Could you check a few things on this model? Use its own coordinates, in mm. A direction names the side the tool comes from. Coordinates: 2 decimals unless noted, no trailing zeros. Loops run counter-clockwise (first coordinate to the right, second up) from the corner with the lowest first, then second, coordinate; pieces in that order, holes last. Notation, with made-up numbers: (51, 45) - (96, 45) arc R25 ccw to (96, 75) - close; hole circle Ø4 at (19, 74). An arc over 180 degrees is marked (long way). One line per question, with ' | ' between items. Start each with the question number.
1. I want a section at C-C, the plane z = 696.5. Write out the boundary of the cut face in (x, y).
2. I'm going to push flat-ended pins straight in: P1, Ø2, axis at x = 12.5, y = 1.5, coming from the +Z side; P2, Ø8, axis at x = -11.5, y = -1, coming from the +Z side. Where does each tip first touch, or does it pass through?
3. I want a section at A-A, the plane x = 4.5. Write out the boundary of the cut face in (y, z).
4. Please list where these lines run through material, in increasing order: L1, parallel to Y at x = -1, z = 61; L2, parallel to Y at x = -13, z = 205. Write a range as [from, to].
5. Which directions (+Z, -Z, +X, -X, +Y, -Y) give clear straight access to the entire face, cutting with the end or side of a thin tool? Please do faces 1 (the flat face through (-14.5, 0, 360)), 2 (the flat face through (17.5, 0, 360)).
6. I want a section at B-B, the plane y = -5. Write out the boundary of the cut face in (x, z).
7. We'd pull the mould along Y, two halves only. Please class faces 3 (the flat face through (0, -17.5, 360)), 4 (the flat face through (14.5, 0, 360)), 5 (the flat face through (0, 15, 730)): pulls with the +Y half, pulls with the -Y half, needs draft (parallel to the pull), parting line crosses it, or undercut.
Autodesk Inventor part; units mm, degrees
ref_plane "Start plane" through (0, 0, -17.5) normal (0, 0, 1) x (1, 0, 0)
ref_plane "End plane" through (0, 0, 747.5) normal (0, 0, 1) x (1, 0, 0)
ref_plane "Work Plane4" through (0, -180, 747.5) normal (0, 0, 1) x (1, 0, 0)
ref_plane "Start plane" through (0, 0, -17.5) normal (0, 0, 1) x (1, 0, 0)
ref_plane "End plane" through (0, 0, 747.5) normal (0, 0, 1) x (1, 0, 0)
sketch "Sketch" plane through (0, 0, 0) normal (0, 0, 1) x (1, 0, 0)
  line L0 (-17.5, -11.5) -> (-17.5, 11.5)
  line L1 (-11.5, 17.5) -> (11.5, 17.5)
  line L2 (17.5, 11.5) -> (17.5, -11.5)
  line L3 (11.5, -17.5) -> (-11.5, -17.5)
  arc A0 (-17.5, -11.5) -> (-11.5, -17.5) centre (-11.5, -11.5) ccw
  arc A1 (-11.5, 17.5) -> (-17.5, 11.5) centre (-11.5, 11.5) ccw
  arc A2 (17.5, 11.5) -> (11.5, 17.5) centre (11.5, 11.5) ccw
  arc A3 (11.5, -17.5) -> (17.5, -11.5) centre (11.5, -11.5) ccw
  arc A4 (-11.5, 14.5) -> (-14.5, 11.5) centre (-11.5, 11.5) ccw
  line L4 (-11.5, 14.5) -> (11.5, 14.5)
  arc A5 (14.5, 11.5) -> (11.5, 14.5) centre (11.5, 11.5) ccw
  line L5 (14.5, 11.5) -> (14.5, -11.5)
  arc A6 (11.5, -14.5) -> (14.5, -11.5) centre (11.5, -11.5) ccw
  line L6 (11.5, -14.5) -> (-11.5, -14.5)
  arc A7 (-14.5, -11.5) -> (-11.5, -14.5) centre (-11.5, -11.5) ccw
  line L7 (-14.5, -11.5) -> (-14.5, 11.5)
  line L8 (0, 25.4278) -> (0, -25.4278) construction
  line L9 (-25.4278, 0) -> (25.4278, 0) construction
  dimension "d7" = 6
  dimension "d10" = 35
  dimension "d11" = 35
  dimension "d12" = 3
  dimension "d15" = 17.5
  dimension "d16" = 17.5
extrude "Body" add sketch "Sketch" along normal up to surface (765 mm away) from surface at -17.5
sketch "Sketch3" plane through (0, 0, 0) normal (0, 0, 1) x (1, 0, 0)
  line L0 (0, 0) -> (10, 0)
ref_plane "Work Plane3" through (0, 0, 0) normal (0, -1, 0) x (1, 0, 0)
sketch "Sketch4" plane through (0, 0, 0) normal (0, -1, 0) x (1, 0, 0)
  line L0 (-2, -17.5) -> (12, -17.5)
  line L1 (-2, 747.5) -> (12, 747.5)
  dimension "d18" = 765
ref_plane "Work Plane4" through (0, -180, 747.5) normal (0, 0, 1) x (1, 0, 0)
split "Split1" plane through (0, -180, 747.5) removes the side toward (0, 0, 1)
ref_plane "Work Plane5" through (0, 0, -17.5) normal (0, 0, -1) x (-1, 0, 0)
split "Split2" plane through (0, 0, -17.5) removes the side toward (0, 0, -1)
ref_plane "Work Plane6" through (-17.5, 0, -17.5) normal (0.7071, 0, -0.7071) x (-0.7071, 0, -0.7071)
split "Split3" plane through (-17.5, 0, -17.5) removes the side toward (0.7071, 0, -0.7071)
ref_plane "Work Plane7" through (-17.5, 0, 747.5) normal (0.7071, 0, 0.7071) x (0.7071, 0, -0.7071)
split "Split4" plane through (-17.5, 0, 747.5) removes the side toward (0.7071, 0, 0.7071)
equation "\"d7\" = G_IR"
equation "\"d10\" = G_H"
equation "\"d11\" = G_W"
equation "\"d12\" = G_T"
equation "\"d15\" = 0.5 * d10"
equation "\"d16\" = 0.5 * d11"
equation "\"d3\" = G_L"
equation "\"G_W\" = 35"
equation "\"G_H\" = 35"
equation "\"G_T\" = 3"
equation "\"G_IR\" = 6"
equation "\"G_L\" = d18"
equation "\"G_OFFSET_START\" = 17.5"
equation "\"G_OFFSET_END\" = 17.5"
equation "\"d13\" = -G_OFFSET_START"
equation "\"d14\" = G_OFFSET_END + B_L"
properties part number "AS 1163 - C350L0 35x35x3.0 SHS - 765" material "Steel, Mild"
Results are:
1) outline: (-17.5, -11.5) arc R6 ccw to (-11.5, -17.5) - (11.5, -17.5) arc R6 ccw to (17.5, -11.5) - (17.5, 11.5) arc R6 ccw to (11.5, 17.5) - (-11.5, 17.5) arc R6 ccw to (-17.5, 11.5) - close; hole (-14.5, -11.5) arc R3 ccw to (-11.5, -14.5) - (11.5, -14.5) arc R3 ccw to (14.5, -11.5) - (14.5, 11.5) arc R3 ccw to (11.5, 14.5) - (-11.5, 14.5) arc R3 ccw to (-14.5, 11.5) - close
2) P1: passes through | P2: stops at z = 745.5
3) outline: (-17.5, 4.5) - (-14.5, 4.5) - (-14.5, 725.5) - (-17.5, 725.5) - close; (14.5, 4.5) - (17.5, 4.5) - (17.5, 725.5) - (14.5, 725.5) - close
4) L1: y = [-17.5, -14.5], [14.5, 17.5] | L2: y = [-17.31, -14.1], [14.1, 17.31]
5) face 1: +Z, -Z | face 2: +Z, -Z, +X, +Y, -Y
6) outline: (-17.5, -17.5) - (-14.5, -14.5) - (-14.5, 744.5) - (-17.5, 747.5) - close; (14.5, 14.5) - (17.5, 17.5) - (17.5, 712.5) - (14.5, 715.5) - close
7) face 3: pulls with the -Y half | face 4: undercut | face 5: needs draft
